Autodesk Inventor part; units mm, degrees
ref_plane "YZ Plane" through (0, 0, 0) normal (1, 0, 0) x (0, 1, 0)
ref_plane "XZ Plane" through (0, 0, 0) normal (0, 1, 0) x (-1, 0, 0)
ref_plane "XY Plane" through (0, 0, 0) normal (0, 0, 1) x (1, 0, 0)
sketch "Sketch1" plane through (0, 0, 0) normal (1, 0, 0) x (0, 1, 0)
  line L0 (25, 27.5) -> (-25, 27.5)
  line L1 (-25, 27.5) -> (-25, -27.5)
  line L2 (-25, -27.5) -> (25, -27.5)
  line L3 (25, -27.5) -> (25, 27.5)
  point P0 (0, 0)
  dimension "d0" = 55
  dimension "d1" = 50
  dimension "d2" = 27.5
  dimension "d3" = 25
extrude "Extrusion1" add sketch "Sketch1" along normal blind 3.175
sketch "Sketch2" plane through (3.175, 0, 0) normal (1, 0, 0) x (0, 0, -1)
  circle A0 centre (-18.25, 9.85) radius 2.5
  circle A1 centre (18.25, 9.85) radius 2.5
  circle A2 centre (-16.5, -16.15) radius 3.175
  circle A3 centre (16.5, -16.15) radius 3.175
  line L0 (27.5, -25) -> (27.5, 25)
  line L1 (-27.5, 25) -> (-27.5, -25)
  line L2 (-27.5, -25) -> (27.5, -25)
  point P0 (0, 0)
  dimension "d6" = 6.35
  dimension "d8" = 11
  dimension "d9" = 11
  dimension "d10" = 6.35
  dimension "d11" = 5
  dimension "d12" = 5
  dimension "d13" = 36.5
  dimension "d14" = 9.25
  dimension "d16" = 8.85
  dimension "d17" = 8.85
  dimension "d22" = 34.85
  dimension "d23" = 34.85
  dimension "d24" = 9.25
extrude "Extrusion2" cut sketch "Sketch2" against normal through all
sketch "Sketch3" plane through (3.175, 0, 0) normal (1, 0, 0) x (0, 0, -1)
  circle A0 centre (0, 9.838) radius 5
  line L0 (27.5, -25) -> (27.5, 25)
  line L1 (27.5, 25) -> (-27.5, 25)
  point P0 (0, 0)
  dimension "d25" = 10
  dimension "d26" = 27.5
  dimension "d27" = 15.162
extrude "Extrusion3" cut sketch "Sketch3" against normal through all
properties part number "BEARING BRACKET MOUNT"
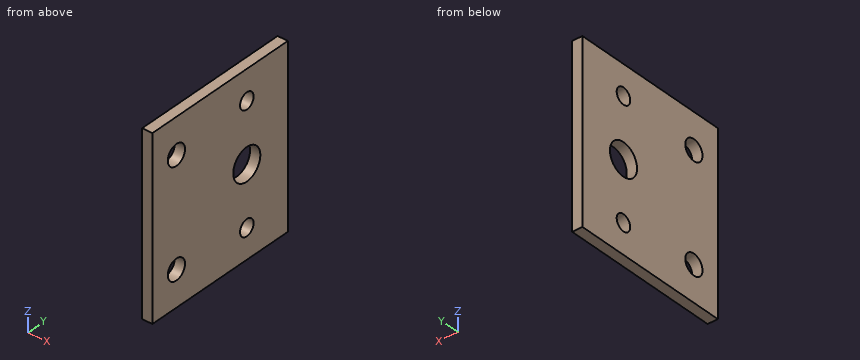
Build history of the part. All positions in model axes, mm. Round coordinates to 2 decimals unless told otherwise and drop trailing zeros. Loops run counter-clockwise (first coordinate to the right, second up) from the corner with the lowest first, then second, coordinate; pieces in that order, holes last. Notation, with made-up numbers: (20, -1.75) -> (29, -1.75) arc R22 cw to (29, 37.25) -> close; hole circle Ø1 at (-10.5, 53.25). An arc over 180 degrees is marked (long way). Use CSV: the item, a comma, the result in double quotes. Start each with the question number.
Q1. Saw through at C-C on z = 16.5. Give the cut face in (x, y) (3 decimals), and give its area (3 significant figures).
Q2. Drill centre lines: L1, parallel to Y at x = 1.45, z = 16.5 (3 decimals); L2, parallel to Z at x = 2.05, y = -19; L3, parallel to Y at x = 1.65, z = -18.25. Where is each one in solid material? Low to high.
Q3. Saw through at D-D on y = 6. Give the cut face in (x, z) (3 decimals).
Q4. Saw through at A-A on z = 0. Give the cut face in (x, y) (3 decimals), and give its area (3 significant figures).
Q5. Saw through at B-B on y = -16.15. Give the cut face in (x, z) (3 decimals).
Q6. Flat gauge pins, fed straight in: pin 1 Ø16 at (y, z) = (9.838, 0) entering from -X; pin 2 Ø3 at (y, z) = (9.85, 18.25) entering from -X. Where does each tip first touch, or does it go through?
Solutions:
1,outline,"(0, -25) -> (3.175, -25) -> (3.175, -19.325) -> (0, -19.325) -> close; (0, -12.975) -> (3.175, -12.975) -> (3.175, 8.065) -> (0, 8.065) -> close; (0, 11.635) -> (3.175, 11.635) -> (3.175, 25) -> (0, 25) -> close"
1,area,"127 mm^2"
2,L1,"y = -25 to -19.325, -12.975 to 8.065, 11.635 to 25"
2,L2,"z = -27.5 to -17.9, -15.1 to 15.1, 17.9 to 27.5"
2,L3,"y = -25 to -18.8, -13.5 to 7.35, 12.35 to 25"
3,outline,"(0, -27.5) -> (3.175, -27.5) -> (3.175, -3.205) -> (0, -3.205) -> close; (0, 3.205) -> (3.175, 3.205) -> (3.175, 27.5) -> (0, 27.5) -> close"
4,outline,"(0, -25) -> (3.175, -25) -> (3.175, 4.838) -> (0, 4.838) -> close; (0, 14.838) -> (3.175, 14.838) -> (3.175, 25) -> (0, 25) -> close"
4,area,"127 mm^2"
5,outline,"(0, -27.5) -> (3.175, -27.5) -> (3.175, -19.675) -> (0, -19.675) -> close; (0, -13.325) -> (3.175, -13.325) -> (3.175, 13.325) -> (0, 13.325) -> close; (0, 19.675) -> (3.175, 19.675) -> (3.175, 27.5) -> (0, 27.5) -> close"
6,pin 1,"stops at x = 0"
6,pin 2,"passes through"
